```python
from build123d import *

# Parameters (mm, degrees)
EXTRUDE1_DEPTH          = 0.3
FILLET1_R               = 0.36
CUT_EXTRUDE1_DEPTH      = 1.3
CUT_EXTRUDE1_DEPTH_BACK = 1.3


with BuildPart() as part:
    # Sketch1 → Extrude1 (new body, symmetric)
    with BuildSketch(Plane(origin=(0, 0, 0), x_dir=(0, 0, -1), z_dir=(1, 0, 0))):
        with BuildLine():
            Line((-2.741249311, -2.094767819), (-0.8428523, -1.36))
            ThreePointArc((-0.8428523, -1.36), (-0.438178046, -1.538830725), (0, -1.6))
            Line((0, -1.6), (0, -2.606451613))
            ThreePointArc((0, -2.606451613), (1.570523601, -2.080155193), (2.506804891, -0.713806172))
            Line((2.506804891, -0.713806172), (1.538830725, -0.438178046))
            ThreePointArc((1.538830725, -0.438178046), (1.6, 0), (1.538830725, 0.438178046))
            Line((1.538830725, 0.438178046), (2.506804891, 0.713806172))
            ThreePointArc((2.506804891, 0.713806172), (1.570523601, 2.080155193), (0, 2.606451613))
            Line((0, 2.606451613), (0, 1.6))
            ThreePointArc((0, 1.6), (-0.438178046, 1.538830725), (-0.8428523, 1.36))
            Line((-0.8428523, 1.36), (-2.741249311, 2.094767819))
            ThreePointArc((-2.741249311, 2.094767819), (3.45, 0), (-2.741249311, -2.094767819))
        make_face()
    extrude(amount=EXTRUDE1_DEPTH, both=True)

    # Fillet1
    fillet1_edges = [part.edges().sort_by_distance(p)[0] for p in [
        (0, -2.094767819, 2.741249311),
        (0, -2.606451613, 0),
        (0, -0.713806172, -2.506804891),
        (0, 0.713806172, -2.506804891),
        (0, 2.606451613, 0),
        (0, 2.094767819, 2.741249311),
    ]]
    fillet(fillet1_edges, radius=FILLET1_R)

    # Sketch4 → Cut-Extrude1 (cut, two sides)
    with BuildSketch(Plane(origin=(0, 0, 0), x_dir=(0, 0, -1), z_dir=(1, 0, 0))) as cut_extrude1_sk:
        with BuildLine():
            ThreePointArc((1.538830725, 0.438178046), (1.584633895, 0.221213517), (1.6, 0))
            ThreePointArc((1.6, 0), (1.721846138, 0.363601628), (2.038178046, 0.580365897))
            Line((2.038178046, 0.580365897), (1.538830725, 0.438178046))
        make_face()
        with BuildLine():
            ThreePointArc((1.6, 0), (1.584633895, -0.221213517), (1.538830725, -0.438178046))
            Line((1.538830725, -0.438178046), (2.038178046, -0.580365897))
            ThreePointArc((2.038178046, -0.580365897), (1.721846138, -0.363601628), (1.6, 0))
        make_face()
    extrude(amount=CUT_EXTRUDE1_DEPTH, mode=Mode.SUBTRACT)
    extrude(cut_extrude1_sk.sketch, amount=-CUT_EXTRUDE1_DEPTH_BACK, mode=Mode.SUBTRACT)


solid = part.part
```
The model under review builds one solid part; all positions refer to its coordinate system, in mm. A direction names the side the tool comes from. Round coordinates to 2 decimals unless told otherwise and drop trailing zeros. Write each loop counter-clockwise with the first axis right and the second up, starting at its lowest first coordinate (ties: lowest second). Pieces come first, ordered by that corner, then holes. Notation, with made-up numbers: (-18, -22.75) - (3, -22.75) arc R21 cw to (3, -16.75) - close; hole circle Ø6 at (87.5, 60.5). An arc over 180 degrees is marked (long way). Use one line per item in the form item = value.
Q1. For line 1 (Y direction, x = -0.05, z = -2); line 2 (Y direction, x = -0.2, z = 1.1); line 3 (Y direction, x = -0.05, z = 2.2), list the stretches that pass through material, from the lowest coordinate up. Write a range as [from, to].
Answer key:
line_1 = [-2.81, -1.67], [-0.57, 0.57], [1.67, 2.81]
line_2 = [-3.27, -1.46], [1.46, 3.27]
line_3 = [-2.66, -1.89], [1.89, 2.66]
Q2. Consider section B-B (x = -0.2). State the section outline as (y, z) points, and give its area (3 significant figures).
Answer key:
outline = (-2.57, -0.42) arc R0.36 cw to (-2.22, 0) - (-1.6, 0) arc R1.6 cw to (-1.36, 0.84) - (-1.91, 2.26) arc R0.36 ccw to (-2.5, 2.37) arc R3.45 ccw (long way) to (2.5, 2.37) arc R0.36 ccw to (1.91, 2.26) - (1.36, 0.84) arc R1.6 cw to (1.6, 0) - (2.22, 0) arc R0.36 cw to (2.57, -0.42) arc R2.61 cw to (1.11, -2.36) arc R0.36 cw to (0.61, -2.13) - (0.58, -2.04) arc R0.6 ccw to (-0.58, -2.04) - (-0.61, -2.13) arc R0.36 cw to (-1.11, -2.36) arc R2.61 cw to start
area = 16.7 mm2
Q3. Consider section D-D (y = 0.5). State the section outline as (x, z) points.
Answer key:
outline = (-0.3, -3.41) - (0.3, -3.41) - (0.3, -1.87) - (-0.3, -1.87) - close
Q4. Consider section A-A (z = -0.55). State the section outline as (x, y) points, and give its area (3 significant figures).
Answer key:
outline = (-0.3, -3.41) - (0.3, -3.41) - (0.3, -2.55) - (-0.3, -2.55) - close; (-0.3, 2.55) - (0.3, 2.55) - (0.3, 3.41) - (-0.3, 3.41) - close
area = 1.03 mm2
Q5. Consider section C-C (z = -1.5). State the section outline as (x, y) points.
Answer key:
outline = (-0.3, -3.11) - (0.3, -3.11) - (0.3, -2.13) - (-0.3, -2.13) - close; (-0.3, 2.13) - (0.3, 2.13) - (0.3, 3.11) - (-0.3, 3.11) - close
Q6. Tool access review of faces 4 (the flat face through (-0.3, 0, -2)), 5 (the cylindrical face through (0.004, 2.069, -1.585)): name each direction out of +Z, -Z, +X, -X, +Y, -Y from which nothing blocks a thin tool from reaching the whole face with its end or side.
Answer key:
face_4 = +Z, -Z, -X, +Y, -Y
face_5 = +X, -X
Q7. Draft analysis for pull direction Y (two halves, no side actions). For faces 1 (the cylindrical face through (0, 0.11, -3.45)), 2 (the flat face through (0.3, 0, -2)), 3 (the cylindrical face through (0, -2.09, -1.56)), state which applies: +Y half, -Y half, draft (parallel to the pull), parting line (faces both ways), or undercut.
Answer key:
face_1 = parting line
face_2 = draft
face_3 = undercut
